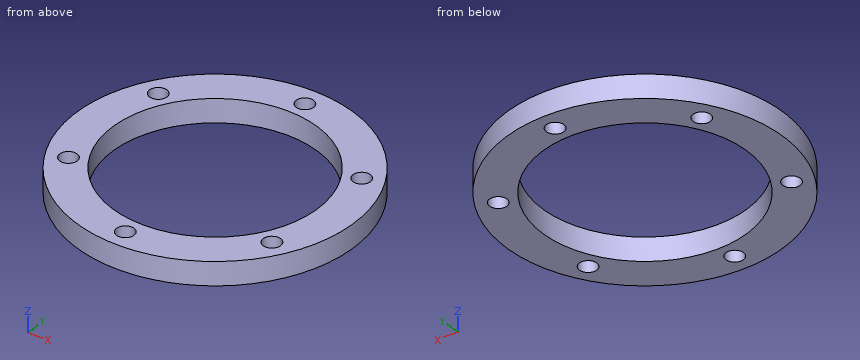
Autodesk Fusion 360 part; units mm, degrees
sketch "Sketch17" plane through (0, 0, 0) normal (0, 0, 1) x (1, 0, 0)
  circle A0 centre (0, 0) radius 26.25
  circle A1 centre (0, 0) radius 35.5
  dimension "d61" = 52.5
  dimension "d62" = 71
extrude "Extrude10" add sketch "Sketch17" along normal blind 6
sketch "Sketch18" plane through (0, 0, 0) normal (0, 0, 1) x (1, 0, 0)
  point P0 (0, 30.5)
sketch "Sketch19" plane through (0, 0, 0) normal (0, 0, 1) x (1, 0, 0)
  circle A0 centre (0, 30.5) radius 2.25
  dimension "d65" = 4.5
extrude "Extrude11" cut sketch "Sketch19" along normal blind 10
pattern_circular "C-Pattern7" count 6 over 360 about axis through (0, 0, 0) along (0, 0, 1) of "Extrude11"
Can you work these out from the model? Positions are in its coordinate system, mm. Round coordinates to 2 decimals unless told otherwise and drop trailing zeros. Loops run counter-clockwise (first coordinate to the right, second up) from the corner with the lowest first, then second, coordinate; pieces in that order, holes last. Notation, with made-up numbers: (29.5, -34) - (46.5, -34) arc R15 ccw to (46.5, -17) - close; hole circle Ø8 at (77, 42). An arc over 180 degrees is marked (long way). Answer in a Markdown table with one row per item. Add a question column.
Q1. I want a section at A-A on x = 0. List the corners of the cut face in (y, z) for me.
Q2. I want a section at C-C on z = 3.85. List the corners of the cut face in (x, y) for me, and give its area (3 significant figures).
Q3. For pin 1 Ø2 at (y, z) = (7, 4) entering from -X; pin 2 Ø1 at (x, z) = (10, 3.5) entering from -Y, each with a flat end and sliding along its axis, tell me the tip position at first contact or that it passes through.
Q4. I need wall thicknesses on L1, parallel to Y at x = 0, z = 1.45; L2, parallel to Y at x = 27, z = 0.8; L3, parallel to X at y = 30.5, z = 4.7. Which ranges of each line are inside material? Lowest first, please.
Q5. I want a section at D-D on x = 21. List the corners of the cut face in (y, z) for me, and give its area (3 significant figures).
Q6. I want a section at B-B on y = 0. List the corners of the cut face in (x, z) for me.
A:
| question | item | result |
|---|---|---|
| 1 | outline | (-35.5, 0) - (-32.75, 0) - (-32.75, 6) - (-35.5, 6) - close; (-28.25, 0) - (-26.25, 0) - (-26.25, 6) - (-28.25, 6) - close; (26.25, 0) - (28.25, 0) - (28.25, 6) - (26.25, 6) - close; (32.75, 0) - (35.5, 0) - (35.5, 6) - (32.75, 6) - close |
| 2 | outline | circle Ø71 at (0, 0); hole circle Ø4.5 at (-26.41, -15.25); hole circle Ø4.5 at (-26.41, 15.25); hole circle Ø52.5 at (0, 0); hole circle Ø4.5 at (0, -30.5); hole circle Ø4.5 at (0, 30.5); hole circle Ø4.5 at (26.41, -15.25); hole circle Ø4.5 at (26.41, 15.25) |
| 2 | area | 1,700 mm^2 |
| 3 | pin 1 | x = -34.99 |
| 3 | pin 2 | y = -34.21 |
| 4 | L1 | -35.5 to -32.75, -28.25 to -26.25, 26.25 to 28.25, 32.75 to 35.5 |
| 4 | L2 | -23.05 to -17.42, -13.08 to 13.08, 17.42 to 23.05 |
| 4 | L3 | -18.17 to -2.25, 2.25 to 18.17 |
| 5 | outline | (-28.62, 0) - (-15.75, 0) - (-15.75, 6) - (-28.62, 6) - close; (15.75, 0) - (28.62, 0) - (28.62, 6) - (15.75, 6) - close |
| 5 | area | 154 mm^2 |
| 6 | outline | (-35.5, 0) - (-26.25, 0) - (-26.25, 6) - (-35.5, 6) - close; (26.25, 0) - (35.5, 0) - (35.5, 6) - (26.25, 6) - close |
